Here's how the part is built. I have some questions about the finished solid (model axes, mm). Face numbers are marked on the shaded views. A direction names the side the tool comes from. Round coordinates to 2 decimals unless told otherwise and drop trailing zeros. Order: outer loops, then holes, each group sorted by start corner. A loop starts at its lowest first (then second) coordinate and runs counter-clockwise, first axis right, second up. Notation, with made-up numbers: (2.25, 48.5) -> (35.25, 48.5) arc R19 cw to (35.25, 57.5) -> close; hole circle Ø8 at (-32, 7). An arc over 180 degrees is marked (long way). Answer in a Markdown table with one row per item.
```python
from build123d import *

# Parameters (mm, degrees)
SKETCH_1_W          = 35
SKETCH_1_H          = 35
EXTRUDE_1_DEPTH     = 40
SKETCH_2_W          = 5.5
SKETCH_2_H          = 5.5
SKETCH_2_H_2        = 4.25
SKETCH_2_W_2        = 4.25
SKETCH_2_W_3        = 3
CUT_EXTRUDE_4_DEPTH = 32.5
SKETCH_3_W          = 5.5
SKETCH_3_H          = 10
CUT_EXTRUDE_5_DEPTH = 3
SKETCH_4_W          = 5.5
SKETCH_4_H          = 10
CUT_EXTRUDE_6_DEPTH = 3
CUT_EXTRUDE_7_DEPTH = 56.957573214
SKETCH_6_W          = 14
SKETCH_6_H          = 35
EXTRUDE_2_DEPTH     = 14
CUT_EXTRUDE_8_DEPTH = 67.687705014
SKETCH_13_R         = 4.1
CUT_EXTRUDE_9_DEPTH = 67.687705014


with BuildPart() as part:
    # Эскиз1 → Бобышка-Вытянуть1 (new body)
    with BuildSketch(Plane.XY):
        Rectangle(SKETCH_1_W, SKETCH_1_H)
    extrude(amount=-EXTRUDE_1_DEPTH)

    # Эскиз2 → Вырез-Вытянуть4 (cut)
    with BuildSketch(Plane.XY):
        Rectangle(SKETCH_2_W, SKETCH_2_H)
        with Locations((0, 4.875)):
            Rectangle(SKETCH_2_W, SKETCH_2_H_2)
        with Locations((0, -4.875)):
            Rectangle(SKETCH_2_W, SKETCH_2_H_2)
        Polygon((10, -10), (10, -2.75), (7, -2.75), (2.75, -2.75), (2.75, -7), (2.75, -10), align=None)
        Polygon((10, 10), (2.75, 10), (2.75, 7), (2.75, 2.75), (7, 2.75), (10, 2.75), align=None)
        Polygon((-2.75, 10), (-10, 10), (-10, 2.75), (-7, 2.75), (-2.75, 2.75), (-2.75, 7), align=None)
        Polygon((-7, -2.75), (-10, -2.75), (-10, -10), (-2.75, -10), (-2.75, -7), (-2.75, -2.75), align=None)
        with Locations((-4.875, 0)):
            Rectangle(SKETCH_2_W_2, SKETCH_2_H)
        with Locations((-8.5, 0)):
            Rectangle(SKETCH_2_W_3, SKETCH_2_H)
        with Locations((4.875, 0)):
            Rectangle(SKETCH_2_W_2, SKETCH_2_H)
        with Locations((8.5, 0)):
            Rectangle(SKETCH_2_W_3, SKETCH_2_H)
    extrude(amount=-CUT_EXTRUDE_4_DEPTH, mode=Mode.SUBTRACT)

    # Эскиз3 → Вырез-Вытянуть5 (cut)
    with BuildSketch(Plane.XZ.offset(-7)):
        with Locations((0, -16.25)):
            Rectangle(SKETCH_3_W, SKETCH_3_H)
    extrude(amount=-CUT_EXTRUDE_5_DEPTH, mode=Mode.SUBTRACT)

    # Эскиз4 → Вырез-Вытянуть6 (cut)
    with BuildSketch(Plane(origin=(0, -7, 0), x_dir=(1, 0, 0), z_dir=(0, 1, 0))):
        with Locations((0, 16.25)):
            Rectangle(SKETCH_4_W, SKETCH_4_H)
    extrude(amount=-CUT_EXTRUDE_6_DEPTH, mode=Mode.SUBTRACT)

    # Эскиз5 → Вырез-Вытянуть7 (cut, through all)
    with BuildSketch(Plane(origin=(0, 17.5, 0), x_dir=(1, 0, 0), z_dir=(0, 1, 0))):
        with BuildLine():
            ThreePointArc((0, 19.1), (-2.85, 16.25), (0, 13.4))
            Line((0, 13.4), (0, 19.1))
        make_face()
        with BuildLine():
            Line((0, 19.1), (0, 13.4))
            ThreePointArc((0, 13.4), (2.015254326, 14.234745674), (2.85, 16.25))
            ThreePointArc((2.85, 16.25), (2.015254326, 18.265254326), (0, 19.1))
        make_face()
    extrude(amount=-CUT_EXTRUDE_7_DEPTH, mode=Mode.SUBTRACT)

    # Эскиз6 → Бобышка-Вытянуть2 (add)
    with BuildSketch(Plane(origin=(0, 0, -40), x_dir=(-1, 0, 0), z_dir=(0, 0, -1))):
        Rectangle(SKETCH_6_W, SKETCH_6_H)
    extrude(amount=EXTRUDE_2_DEPTH)

    # Эскиз7 → Вырез-Вытянуть8 (cut, through all)
    with BuildSketch(Plane(origin=(0, 17.5, 0), x_dir=(1, 0, 0), z_dir=(0, 1, 0))):
        with BuildLine():
            ThreePointArc((0, 51.03), (-4.03, 47), (0, 42.97))
            Line((0, 42.97), (0, 51.03))
        make_face()
        with BuildLine():
            Line((0, 51.03), (0, 42.97))
            ThreePointArc((0, 42.97), (2.849640328, 44.150359672), (4.03, 47))
            ThreePointArc((4.03, 47), (2.849640328, 49.849640328), (0, 51.03))
        make_face()
    extrude(amount=-CUT_EXTRUDE_8_DEPTH, mode=Mode.SUBTRACT)

    # Эскиз13 → Вырез-Вытянуть9 (cut, through all)
    with BuildSketch(Plane.XZ.offset(17.5)):
        with Locations(Location((0, -47, 0), (0, 0, 270))):
            Circle(SKETCH_13_R)
    extrude(amount=-CUT_EXTRUDE_9_DEPTH, mode=Mode.SUBTRACT)


solid = part.part
```
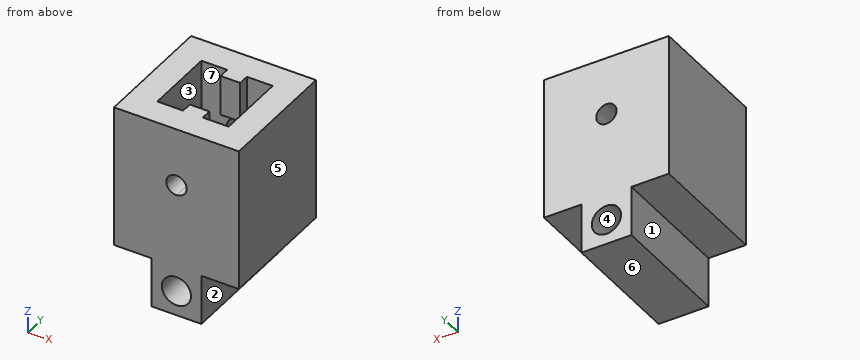
1. Please list where these lines run through material, in increasing order: line 1 along X through (y, z) = (-5, -47); line 2 along Y through (x, z) = (5.5, -17); line 3 along Z through (x, y) = (-1, -9.5).
Numbers:
| item | result |
|---|---|
| line 1 | x = -7 to -4.1, 4.1 to 7 |
| line 2 | y = -17.5 to -10, 10 to 17.5 |
| line 3 | z = -54 to -50.98, -43.02 to -21.25, -11.25 to 0 |
2. Suppose I cut it at B-B on z = -47. Write out the boundary of the cut face in (x, y).
Numbers:
| item | result |
|---|---|
| outline | (-7, -17.5) -> (-4.1, -17.5) -> (-4.1, 17.5) -> (-7, 17.5) -> close; (4.1, -17.5) -> (7, -17.5) -> (7, 17.5) -> (4.1, 17.5) -> close |
3. For pin 1 Ø11 at (y, z) = (-7.5, -47.5) entering from +X; pin 2 Ø8.5 at (x, y) = (-14, -2.5) entering from -Z; pin 3 Ø3.5 at (x, y) = (-1, -8.5) entering from +Z; pin 4 Ø11 at (y, z) = (3, -50) entering from -X, each with a flat end and sliding along its axis, tell me the tip position at first contact or that it passes through.
Numbers:
| item | result |
|---|---|
| pin 1 | stops at x = 7 |
| pin 2 | stops at z = -40 |
| pin 3 | stops at z = 0 |
| pin 4 | stops at x = -7 |
4. Suppose I cut it at D-D on y = 2.5. Write out the boundary of the cut face in (x, z).
Numbers:
| item | result |
|---|---|
| outline | (-17.5, -40) -> (-7, -40) -> (-7, -54) -> (7, -54) -> (7, -40) -> (17.5, -40) -> (17.5, 0) -> (10, 0) -> (10, -32.5) -> (-10, -32.5) -> (-10, 0) -> (-17.5, 0) -> close; hole circle Ø8.2 at (0, -47) |
5. We'd pull the mould along X, two halves only. Please class the marked faces 4, 5, 6 and 7: released by +X, released by -X, zero draft, split by the parting line, or undercut.
Numbers:
| item | result |
|---|---|
| face 4 | undercut |
| face 5 | released by +X |
| face 6 | zero draft |
| face 7 | undercut |
6. For the marked faces 1, 2 and 3, which set-ups out of +Z, -Z, +X, -X, +Y, -Y let a thin tool reach every point of the face, with its end or its side?
Numbers:
| item | result |
|---|---|
| face 1 | -Z, -X, +Y, -Y |
| face 2 | -Z, +X, +Y, -Y |
| face 3 | +Z |
7. Suppose I cut it at C-C on z = -29. Write out the boundary of the cut face in (x, y).
Numbers:
| item | result |
|---|---|
| outline | (-17.5, -17.5) -> (17.5, -17.5) -> (17.5, 17.5) -> (-17.5, 17.5) -> close; hole (-10, -10) -> (-2.75, -10) -> (-2.75, -7) -> (2.75, -7) -> (2.75, -10) -> (10, -10) -> (10, 10) -> (2.75, 10) -> (2.75, 7) -> (-2.75, 7) -> (-2.75, 10) -> (-10, 10) -> close |
8. Suppose I cut it at A-A on y = 15.5. Write out the boundary of the cut face in (x, z), then the cut area to 3 significant figures.
Numbers:
| item | result |
|---|---|
| outline | (-17.5, -40) -> (-7, -40) -> (-7, -54) -> (7, -54) -> (7, -40) -> (17.5, -40) -> (17.5, 0) -> (-17.5, 0) -> close; hole circle Ø8.2 at (0, -47); hole circle Ø5.7 at (0, -16.25) |
| area | 1,520 mm2 |
